The model under review builds one solid part; all positions refer to its coordinate system, in mm. Give positions to 0.01 mm unless a question says otherwise; leave off trailing zeros. Loops run counter-clockwise (first coordinate to the right, second up) from the corner with the lowest first, then second, coordinate; pieces in that order, holes last. Notation, with made-up numbers: M 12,62.5 L 54,62.5 A22 ccw 54,79.5 Z; hole C 21,-7.5 d11. An arc over 180 degrees is marked long. Return JSON: item names as keys, results as strings. Group by question number.
```python
from build123d import *

# Parameters (mm, degrees)
TORUS_R        = 8
TORUS001_R     = 8
CYLINDER_R     = 50
CYLINDER_DEPTH = 10


with BuildPart() as obj1:
    # Torus → Torus (revolve)
    with BuildSketch(Plane(origin=(0, 0, 9), x_dir=(1, 0, 0), z_dir=(0, -1, 0))):
        with Locations((20, 0)):
            Circle(TORUS_R)
    revolve(axis=Axis((0, 0, 9), (0, 0, 1)))


with BuildPart() as obj2:
    # Torus001 → Torus001 (revolve)
    with BuildSketch(Plane(origin=(0, 0, 9), x_dir=(1, 0, 0), z_dir=(0, -1, 0))):
        with Locations((40, 0)):
            Circle(TORUS001_R)
    revolve(axis=Axis((0, 0, 9), (0, 0, 1)))

    # Fusion: union obj1
    add(obj1.part)


with BuildPart() as obj3:
    # Cylinder → Cylinder (new body)
    with BuildSketch(Plane.XY):
        Circle(CYLINDER_R)
    extrude(amount=CYLINDER_DEPTH)

    # Cut: cut obj2
    add(obj2.part, mode=Mode.SUBTRACT)


solid = obj3.part
```
(1) Add section B-B (y = 0). Write out the cut boundary in (x, z).
(2) For pin 1 (6 mm diameter, centred on y = 29.5, z = 3, fed in from +X); pin 2 (10 mm diameter, centred on x = -18, y = -32, fed in from -Z); pin 3 (6 mm diameter, centred on x = 32.5, z = 6.5, fed in from -Y); pin 4 (2 mm diameter, centred on x = -26, z = 3.5, fed in from +Y), all flat-tipped, find the tip position at first contact; note any pin that passes through.
(3) Add section A-A (z = 7.5). Write out the cut boundary in (x, y).
(4) For probe 1 along Y at (x, z) = (-23, 4); probe 2 along X at (y, z) = (-29, 9.5); probe 3 along X at (y, z) = (7.5, 1.75), list the stretches that pass through material, from the lowest coordinate up.
Verdict:
{
 "1": {"outline": "M -50,0 L 50,0 L 50,10 L 47.94,10 A8 cw long 32.06,10 L 27.94,10 A8 cw long 12.06,10 L -12.06,10 A8 cw long -27.94,10 L -32.06,10 A8 cw long -47.94,10 L -50,10 Z"},
 "2": {"pin 1": "stops at x = 42.4", "pin 2": "stops at z = 0", "pin 3": "stops at y = -40.37", "pin 4": "stops at y = 43.3"},
 "3": {"outline": "C 0,0 d100; C 0,0 d64.28; C 0,0 d24.28; hole C 0,0 d95.72; hole C 0,0 d55.72"},
 "4": {"probe 1": "y = -44.4 to -40.12, -24.71 to -12.64, 12.64 to 24.71, 40.12 to 44.4", "probe 2": "x = -40.73 to -38.23, -13.56 to 13.56, 38.23 to 40.73", "probe 3": "x = -49.43 to -42.73, -35.84 to -22.15, -14.83 to 14.83, 22.15 to 35.84, 42.73 to 49.43"}
}
